Read the model definition and answer for the solid it produces. Units are mm, in the model's axes. Face numbers are marked on the shaded views. A direction names the side the tool comes from. Give positions to 0.01 mm unless a question says otherwise; leave off trailing zeros. Write each loop counter-clockwise with the first axis right and the second up, starting at its lowest first coordinate (ties: lowest second). Pieces come first, ordered by that corner, then holes. Notation, with made-up numbers: M 71,63 L 75,63 A25 ccw 75,81 Z; hole C 0,29.5 d2. An arc over 180 degrees is marked long. Put each result on its own line as item: value.
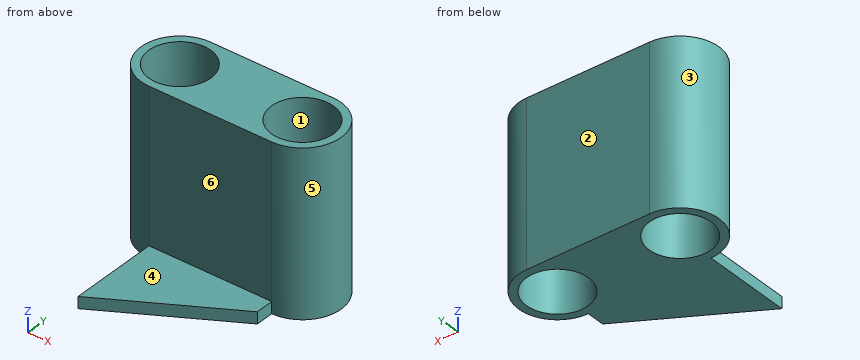
from build123d import *

# Parameters (mm, degrees)
F0_R     = 8
F1_DEPTH = 42.3
F2_W     = 31.75
F2_H     = 23
F3_DEPTH = 3
F5_DEPTH = 25


with BuildPart() as f1:
    # F0 (on Top) → F1 (new body)
    with BuildSketch(Plane.XY):
        with BuildLine():
            Line((-15.875, -10), (15.875, -10))
            ThreePointArc((15.875, -10), (25.875, 0), (15.875, 10))
            Line((15.875, 10), (-15.875, 10))
            ThreePointArc((-15.875, 10), (-25.875, 0), (-15.875, -10))
        make_face()
        with Locations((-15.875, 0)):
            Circle(F0_R, mode=Mode.SUBTRACT)
        with Locations((15.875, 0)):
            Circle(F0_R, mode=Mode.SUBTRACT)
    extrude(amount=F1_DEPTH)

    # F2 (on Top) → F3 (join)
    with BuildSketch(Plane.XY):
        with Locations((0, -21.5)):
            Rectangle(F2_W, F2_H)
    extrude(amount=F3_DEPTH)

    # F4 (on face) → F5 (cut)
    with BuildSketch(Plane(origin=(0, 0, 0), x_dir=(1, 0, 0), z_dir=(0, 0, -1))):
        Polygon((15.875, 33), (-15.875, 33), (15.875, 14.669129), align=None)
    extrude(amount=-F5_DEPTH, mode=Mode.SUBTRACT)


solid = f1.part
(1) Which of the six approach directions +Z, -Z, +X, -X, +Y, -Y give full straight-line access (tool end or side, diameter ignored) to the marked faces 5 and 6?
Result:
face 5: +Z, -Z, +X
face 6: +Z, +X, -X, -Y
(2) Section A-A on z = 19 is taken. Determine the outline of the cut face in (x, y) (3 decimals), and give its area (3 significant figures).
Result:
outline: M -15.875,-10 L 15.875,-10 A10 ccw 15.875,10 L -15.875,10 A10 ccw Z; hole C -15.875,0 d16; hole C 15.875,0 d16
area: 547 mm²
(3) Section D-D on y = -7 is taken. Determine the outline of the cut face in (x, z), and give its area (3 significant figures).
Result:
outline: M -23.02,0 L -19.75,0 L -19.75,42.3 L -23.02,42.3 Z; M -12,0 L 12,0 L 12,42.3 L -12,42.3 Z; M 19.75,0 L 23.02,0 L 23.02,42.3 L 19.75,42.3 Z
area: 1,290 mm²
(4) Straight lines are drawn through the part: line 1 along X through (y, z) = (-7, 2); line 2 along X through (y, z) = (4, 27); line 3 along Z through (x, y) = (-15.5, -28.5). For each, find the intervals that lie inside material, in ascending order. Write a range as from..to.
Result:
line 1: x = -23.02..-19.75, -12..12, 19.75..23.02
line 2: x = -25.04..-22.8, -8.95..8.95, 22.8..25.04
line 3: z = 0..3
(5) Section C-C on y = 0 is taken. Determine the outline of the cut face in (x, z) (3 decimals).
Result:
outline: M -25.875,0 L -23.875,0 L -23.875,42.3 L -25.875,42.3 Z; M -7.875,0 L 7.875,0 L 7.875,42.3 L -7.875,42.3 Z; M 23.875,0 L 25.875,0 L 25.875,42.3 L 23.875,42.3 Z
(6) For a pull along Y with two mould halves and no side action, classify the marked faces 1, 2, 3 and 4 as +Y half, -Y half, draft (parallel to the pull), parting line (faces both ways), or undercut.
Result:
face 1: undercut
face 2: +Y half
face 3: parting line
face 4: draft
(7) Section B-B on x = 13 is taken. Determine the outline of the cut face in (y, z), and give its area (3 significant figures).
Result:
outline: M -16.33,0 L -7.47,0 L -7.47,42.3 L -10,42.3 L -10,3 L -16.33,3 Z; M 7.47,0 L 10,0 L 10,42.3 L 7.47,42.3 Z
area: 233 mm²
(8) Given pin 1 Ø1 at (y, z) = (-1.5, 37.5) entering from -X; pin 2 Ø2 at (x, z) = (-5.5, 15) entering from -Y; pin 3 Ø7 at (x, y) = (1.5, -25.5) entering from +Z, each flat-ended and moving along its own axis, determine where each tip first touches the part or whether it passes through.
Result:
pin 1: stops at x = -25.82
pin 2: stops at y = -10
pin 3: stops at z = 3
